```python
from build123d import *

# Parameters (mm, degrees)
BOSS_EXTRUDE2_DEPTH = 5
CUT_EXTRUDE1_DEPTH  = 5
CUT_EXTRUDE2_DEPTH  = 5
SKETCH7_R           = 2.5
CUT_EXTRUDE3_DEPTH  = 5


with BuildPart() as part:
    # Sketch4 → Boss-Extrude2 (new body)
    with BuildSketch(Plane.XY):
        with BuildLine():
            Line((0, 10), (20, 10))
            Line((20, 10), (26.307466479, 0.203296746))
            Line((26.307466479, 0.203296746), (15.504252616, 0))
            Line((15.504252616, 0), (0, 0))
            ThreePointArc((0, 0), (-5, 5), (0, 10))
        make_face()
    extrude(amount=BOSS_EXTRUDE2_DEPTH)

    # Sketch5 → Cut-Extrude1 (cut)
    with BuildSketch(Plane.XY.offset(5)):
        Polygon((6.379128738, 0), (9.016156307, 3.359284814), (19.402963043, 3.359284814), (20.614889369, 0.096172846), align=None)
    extrude(amount=-CUT_EXTRUDE1_DEPTH, mode=Mode.SUBTRACT)

    # Sketch6 → Cut-Extrude2 (cut)
    with BuildSketch(Plane(origin=(0, 0, 0), x_dir=(-1, 0, 0), z_dir=(0, 0, -1))):
        Polygon((-20.614889369, 0.096172846), (-6.379128738, 0), (-6.379128738, -1.250967918), (-21.241056997, -1.250967918), align=None)
    extrude(amount=-CUT_EXTRUDE2_DEPTH, mode=Mode.SUBTRACT)

    # Sketch7 → Cut-Extrude3 (cut)
    with BuildSketch(Plane(origin=(0, 0, 0), x_dir=(-1, 0, 0), z_dir=(0, 0, -1))):
        with Locations((0, 5.324946676)):
            Circle(SKETCH7_R)
    extrude(amount=-CUT_EXTRUDE3_DEPTH, mode=Mode.SUBTRACT)


solid = part.part
```
CAD build for the part. Positions are in the model's coordinates, mm. A direction names the side the tool comes from. Give positions to 0.01 mm unless a question says otherwise; leave off trailing zeros. Write each loop counter-clockwise with the first axis right and the second up, starting at its lowest first coordinate (ties: lowest second). Pieces come first, ordered by that corner, then holes. Notation, with made-up numbers: M 81.25,82.25 L 111.25,82.25 A34 ccw 111.25,116.25 Z; hole C 12,48.5 d10. An arc over 180 degrees is marked long. Return JSON: item names as keys, results as strings. Group by question number.
(1) 3-axis set-ups, long thin cutter, end or side, ignore diameter. For faces 1 (the face through (14, 3.359, 3)), 2 (the face through (-5, 5, 2)): which of +Z, -Z, +X, -X, +Y, -Y reach the whole face in a straight line?
(2) Flat gauge pins, fed straight in: pin 1 Ø1 at (x, z) = (22, 1.5) entering from -Y; pin 2 Ø4 at (x, y) = (0, 5.32) entering from +Z; pin 3 Ø1 at (x, z) = (17.5, 1) entering from -Y; pin 4 Ø3 at (y, z) = (8.5, 4) entering from -X. Where does each tip first touch, or does it go through?
(3) Band-saw the part on D-D (x = 12.5). Give the cut face in (y, z).
(4) Band-saw the part on A-A (z = 3.8). Give the cut face in (x, y).
(5) Band-saw the part on C-C (x = -2). Give the cut face in (y, z), and give its area (3 significant figures).
(6) Mould opens along X. For faces 3 (the face through (23.11, 5.17, 2.46)), 4 (the face through (0.542, 2.884, 2.465)), 5 (the face through (10, 10, 2)) say: pulls with the +X half, pulls with the -X half, needs draft (parallel to the pull), parting line crosses it, or undercut.
(7) Drill centre lines: L1, parallel to Y at x = 0, z = 3.4; L2, parallel to Y at x = 12, z = 0.6; L3, parallel to Y at x = 0.5, z = 2.35. Where is each one in solid material? Low to high. Write a range as [from, to].
(8) Band-saw the part on B-B (y = 5). Give the cut face in (x, z).
Entries:
{
 "1": {"face 1": "+Z, -Z, -Y", "face 2": "+Z, -Z, -X"},
 "2": {"pin 1": "stops at y = 0.11", "pin 2": "passes through", "pin 3": "stops at y = 3.36", "pin 4": "stops at x = -4.58"},
 "3": {"outline": "M 3.36,0 L 10,0 L 10,5 L 3.36,5 Z"},
 "4": {"outline": "M 0,0 L 6.38,0 L 9.02,3.36 L 19.4,3.36 L 20.61,0.1 L 26.31,0.2 L 20,10 L 0,10 A5 ccw Z; hole C 0,5.32 d5"},
 "5": {"outline": "M 0.42,0 L 3.82,0 L 3.82,5 L 0.42,5 Z; M 6.82,0 L 9.58,0 L 9.58,5 L 6.82,5 Z", "area": "30.8 mm^2"},
 "6": {"face 3": "pulls with the +X half", "face 4": "undercut", "face 5": "needs draft"},
 "7": {"L1": "y = [0, 2.82], [7.82, 10]", "L2": "y = [3.36, 10]", "L3": "y = [0, 2.88], [7.77, 10]"},
 "8": {"outline": "M -5,0 L -2.48,0 L -2.48,5 L -5,5 Z; M 2.48,0 L 23.22,0 L 23.22,5 L 2.48,5 Z"}
}
